Can you work these out from the model? Positions are in its coordinate system, mm. Face numbers are marked on the shaded views. A direction names the side the tool comes from. Give positions to 0.01 mm unless a question says otherwise; leave off trailing zeros. Order: outer loops, then holes, each group sorted by start corner. A loop starts at its lowest first (then second) coordinate and runs counter-clockwise, first axis right, second up. Notation, with made-up numbers: (49, 20.25) -> (67, 20.25) arc R28 cw to (67, 52.25) -> close; hole circle Ø11 at (25.25, 47). An arc over 180 degrees is marked (long way). Answer as CSV lines item,"result".
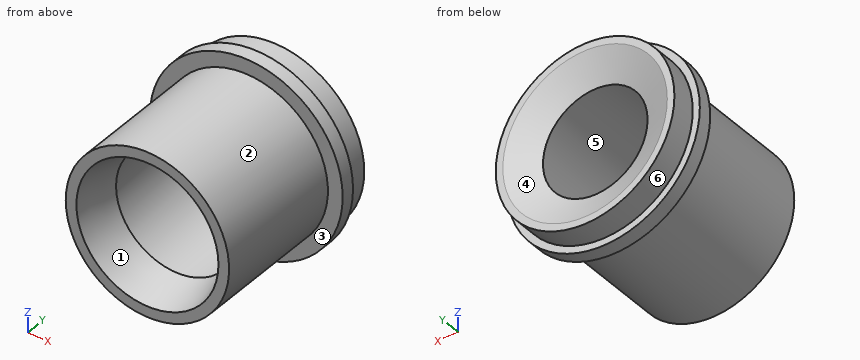
Autodesk Inventor part; units mm, degrees
ref_plane "YZ Plane" through (0, 0, 0) normal (1, 0, 0) x (0, 1, 0)
ref_plane "XZ Plane" through (0, 0, 0) normal (0, 1, 0) x (-1, 0, 0)
ref_plane "XY Plane" through (0, 0, 0) normal (0, 0, 1) x (1, 0, 0)
sketch "Sketch1" plane through (0, 0, 0) normal (0, 0, 1) x (1, 0, 0)
  line L0 (0, 25.4) -> (-28.702, 25.4) construction
  line L1 (0, 25.4) -> (-86.36, 25.4) construction
  line L2 (-86.36, 25.4) -> (-80.01, 25.4) construction
  line L3 (-80.01, 25.4) -> (-73.66, 22.4389) construction
  line L4 (-80.01, 25.4) -> (-80.01, 22.4389) construction
  line L5 (-80.01, 0) -> (-86.36, 0)
  line L6 (-28.702, 59.6457) -> (-28.702, -91.9304) construction
  arc A0 (-28.9184, -4.2142) -> (-32.3684, 3.1843) centre (-35.052, -2.5707) ccw
  line L7 (-67.31, -147.4937) -> (-28.9184, -4.2142)
  line L8 (-80.01, 22.4389) -> (-73.66, 22.4389)
  line L9 (-80.01, 22.4389) -> (-80.01, 0)
  line L10 (-73.66, 22.4389) -> (-32.3684, 3.1843)
  line L11 (-28.702, -2.5707) -> (-60.452, -2.5707) construction
  line L12 (-60.452, 16.28) -> (-60.452, -121.8993) construction
  line L13 (-60.452, -121.8993) -> (-54.102, -121.8993) construction
  line L14 (-54.102, -121.8993) -> (-54.102, -98.2008) construction
  line L15 (-54.102, -98.2008) -> (-60.452, -98.2008)
  line L16 (-60.452, 16.28) -> (-60.452, 6.755) construction
  line L17 (-60.452, 16.28) -> (-60.452, 9.93) construction
  line L18 (-60.452, 9.93) -> (-46.8344, 9.93)
  line L19 (-60.452, 9.93) -> (-60.452, -98.2008)
  line L20 (-86.36, 0) -> (-86.36, -12.7) construction
  line L21 (-60.452, -12.7) -> (-73.152, -12.7) construction
  line L22 (-86.36, -12.7) -> (-86.36, -25.4) construction
  line L23 (-86.36, -25.4) -> (-86.36, -88.9) construction
  line L24 (-86.36, -88.9) -> (-73.66, -88.9) construction
  line L25 (-73.66, -88.9) -> (-73.66, -25.4) construction
  line L26 (-86.36, -25.4) -> (-73.66, -25.4)
  line L27 (-73.66, -25.4) -> (-73.66, -88.9)
  line L28 (-73.66, -88.9) -> (-86.36, -88.9)
  line L29 (-86.36, -12.7) -> (-73.152, -12.7)
  line L30 (-73.152, -133.7486) -> (-63.627, -133.7486)
  line L31 (-73.66, -88.9) -> (-73.66, -147.4937)
  line L32 (-73.66, -147.4937) -> (-67.31, -147.4937)
  line L33 (-73.152, -12.7) -> (-73.152, -133.7486)
  line L34 (-80.01, -25.4) -> (-80.01, -31.3436)
  line L35 (-80.01, -31.3436) -> (-86.36, -31.3436)
  line L36 (-86.36, 0) -> (-86.36, -25.4)
  line L37 (-86.36, -31.3436) -> (-86.36, -88.9)
  line L38 (0, -319.0244) -> (0, 122.7573)
  point P0 (0, 0)
  point P1 (-86.36, -255.9127)
  point P2 (-76.835, 22.4389)
  dimension "d0" = 28.702
  dimension "d1" = 86.36
  dimension "d2" = 6.35
  dimension "d3" = 25
  dimension "d5" = 25.4
  dimension "d6" = 25.4
  dimension "d8" = 12.7
  dimension "d11" = 6.35
  dimension "d12" = 31.75
  dimension "d13" = 6.35
  dimension "d15" = 6.35
  dimension "d16" = 12.7
  dimension "d17" = 12.7
  dimension "d18" = 12.7
  dimension "d19" = 63.5
  dimension "d20" = 12.7
  dimension "d22" = 9.525
  dimension "d23" = 6.35
  dimension "d25" = 5.9436
  dimension "d26" = 15
revolve "Revolution2" add sketch "Sketch1" angle 360 about axis through (0, -10, 0) along (0, 1, 0) contours L9 L8 L10 L18 L19 L15 L7 L30 L33 L29 L36 L5
properties part number "Phenolic Master Sketch" material "Phenolic Resin"
Item 1: Imagine slicing it at A-A, the plane x = 0. Please give me the cut outline in (y, z).
Numbers:
outline,"(-133.75, -73.15) -> (-12.7, -73.15) -> (-12.7, -86.36) -> (0, -86.36) -> (0, -80.01) -> (22.44, -80.01) -> (22.44, -73.66) -> (9.93, -46.83) -> (9.93, -60.45) -> (-98.2, -60.45) -> (-98.2, -54.1) -> (-133.75, -63.63) -> close; (-133.75, 63.63) -> (-98.2, 54.1) -> (-98.2, 60.45) -> (9.93, 60.45) -> (9.93, 46.83) -> (22.44, 73.66) -> (22.44, 80.01) -> (0, 80.01) -> (0, 86.36) -> (-12.7, 86.36) -> (-12.7, 73.15) -> (-133.75, 73.15) -> close"
Item 2: Please list where these lines run through material, in increasing order: line 1 along Z through (x, y) = (0, -75.5); line 2 along Z through (x, y) = (50, -65.5); line 3 along X through (y, z) = (-72, 40.5).
Numbers:
line 1,"z = -73.15 to -60.45, 60.45 to 73.15"
line 2,"z = -53.4 to -33.98, 33.98 to 53.4"
line 3,"x = -60.92 to -44.88, 44.88 to 60.92"
Item 3: For the marked faces 5 and 6, which set-ups out of +Z, -Z, +X, -X, +Y, -Y let a thin tool reach every point of the face, with its end or its side?
Numbers:
face 5,"none"
face 6,"+Y"
Item 4: Imagine slicing it at B-B, the plane z = 0. Please give me the cut outline in (x, y).
Numbers:
outline,"(-86.36, -12.7) -> (-73.15, -12.7) -> (-73.15, -133.75) -> (-63.63, -133.75) -> (-54.1, -98.2) -> (-60.45, -98.2) -> (-60.45, 9.93) -> (-46.83, 9.93) -> (-73.66, 22.44) -> (-80.01, 22.44) -> (-80.01, 0) -> (-86.36, 0) -> close; (46.83, 9.93) -> (60.45, 9.93) -> (60.45, -98.2) -> (54.1, -98.2) -> (63.63, -133.75) -> (73.15, -133.75) -> (73.15, -12.7) -> (86.36, -12.7) -> (86.36, 0) -> (80.01, 0) -> (80.01, 22.44) -> (73.66, 22.44) -> close"
Item 5: Imagine slicing it at C-C, the plane y = -19.5. Please give me the cut outline in (x, z).
Numbers:
outline,"circle Ø146.3 at (0, 0); hole circle Ø120.9 at (0, 0)"
Item 6: For pin 1 (6 mm diameter, centred on x = -5.5, y = -92, fed in from +Z); pin 2 (3 mm diameter, centred on y = -35.5, z = -64.5, fed in from -X); pin 3 (8 mm diameter, centred on y = -2, z = -6.5, fed in from -X), each with a flat end and sliding along its axis, tell me the tip position at first contact or that it passes through.
Numbers:
pin 1,"stops at z = 73.11"
pin 2,"stops at x = -37.18"
pin 3,"stops at x = -86.32"
Item 7: We'd pull the mould along Z, two halves only. Please class the marked faces 1, 2, 3 and 4: released by +Z, released by -Z, zero draft, split by the parting line, or undercut.
Numbers:
face 1,"undercut"
face 2,"split by the parting line"
face 3,"zero draft"
face 4,"undercut"
